Part model, mm, in its own coordinate system. Face numbers are marked on the shaded views. A direction names the side the tool comes from. Round coordinates to 2 decimals unless told otherwise and drop trailing zeros. Use CSV: the item, a comma, the result in double quotes. Start each with the question number.
(1) Drop flat-ended pins along their axis: pin 1 (5 mm diameter, centred on x = 94, z = 2, fed in from +Y); pin 2 (1.5 mm diameter, centred on y = -3, z = 3.5, fed in from +X); pin 3 (1 mm diameter, centred on x = 35, z = 4.5, fed in from -Y). Give the stop position or say it passes through.
(2) Which spindle directions (+Z, -Z, +X, -X, +Y, -Y) get a long thin tool onto all of the face, cutting with end or side? Do the marked faces 1 and 2. Say none if no direction does.
(3) Probe line 1 (X direction, y = -1.75, z = 6.25); line 2 (Y direction, x = 25.5, z = 0.25); line 3 (Y direction, x = 120, z = 0.25). List the from-to ranges inside material, lowest first. Write a range as [from, to].
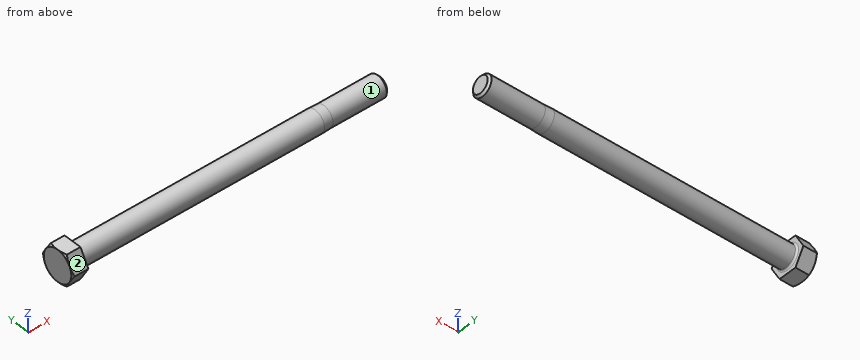
Autodesk Inventor part; units mm, degrees
ref_plane "Work Plane1" through (1.525, 0, 0) normal (0, 0, 1) x (1, 0, 0)
ref_plane "YZ Plane" through (0, 0, 0) normal (1, 0, 0) x (0, 1, 0)
ref_plane "XZ Plane" through (0, 0, 0) normal (0, 1, 0) x (-1, 0, 0)
sketch "Sketch1" plane through (0, 0, 0) normal (0, 0, 1) x (1, 0, 0)
  line L0 (0, 7.1374) -> (0, 4.9276)
  line L1 (114.3, 4.7625) -> (139.7, 4.7625)
  line L2 (139.7, 4.7625) -> (139.7, 0)
  line L3 (139.7, 0) -> (-0.0001, 0)
  line L4 (-27.9401, 0) -> (167.64, 0)
  line L5 (-0.0001, 0) -> (-0.0001, 7.1374)
  line L6 (-0.0001, 7.1374) -> (0, 7.1374)
  line L7 (114.3, 4.7625) -> (110.3312, 4.9276)
  line L8 (110.3312, 4.9276) -> (0, 4.9276)
  line L9 (0, -1.4275) -> (0, 8.5649)
  dimension "d0" = 139.7
  dimension "d1" = 25.4
  dimension "d2" = 9.525
  dimension "d9" = 0.0001
  dimension "d10" = 14.2748
  dimension "d13" = 3.9689
  dimension "d14" = 9.8552
revolve "Body" add sketch "Sketch1" angle 360 about axis through (139.7, 0, 0) along (-1, 0, 0)
sketch "Sketch2" plane through (-0.0001, 0, 0) normal (-1, 0, 0) x (0, 0, 1)
  line L0 (0, 8.2416) -> (7.1374, 4.1208)
  line L1 (7.1374, 4.1208) -> (7.1374, -4.1208)
  line L2 (7.1374, -4.1208) -> (0, -8.2416)
  line L3 (0, -8.2416) -> (-7.1374, -4.1208)
  line L4 (-7.1374, -4.1208) -> (-7.1374, 4.1208)
  line L5 (-7.1374, 4.1208) -> (0, 8.2416)
  point P0 (0, 0)
  point P1 (0, 0)
  dimension "d11" = 14.2748
extrude "Head" add sketch "Sketch2" along normal blind 6.8072
sketch "Sketch4" plane through (0, 0, 0) normal (0, 0, 1) x (1, 0, 0)
  line L0 (-6.8073, 7.1374) -> (-6.8073, 8.2416)
  line L1 (-6.8073, 8.2416) -> (-6.1698, 8.2416)
  line L2 (-6.1698, 8.2416) -> (-6.8073, 7.1374)
  line L3 (-8.1687, 0) -> (1.3613, 0)
  line L4 (-0.0001, 8.2416) -> (-6.8073, 8.2416)
  line L5 (-6.8073, 4.1208) -> (-6.8073, 8.2416)
  dimension "d5" = 30
  dimension "d19" = 14.2748
revolve "Chamfer1" cut sketch "Sketch4" angle 360 about axis through (-10, 0, 0) along (1, 0, 0)
thread "Thread"
chamfer "Chamfer2" distance 0.9739 distance2 0.9447 1 edges at (139.7, -4.7625, 0) measured on face at (139.7, -0.9018, 0.7989)
ref_plane "Work Plane1" through (1.525, 0, 0) normal (0, 0, 1) x (1, 0, 0)
fillet "Fillet2" radius 0.762 1 edges at (0, -4.9276, 0)
equation "\"d0\" = NLG"
equation "\"d1\" = GEL"
equation "\"d2\" = GD"
equation "\"d10\" = SD2"
equation "\"d14\" = BDM"
equation "\"d11\" = SW"
equation "\"d3\" = KOH - SD"
equation "\"d5\" = ANG1"
equation "\"d19\" = SW0"
equation "\"d63\" = R"
equation "\"d15\" = GEL"
equation "\"d6\" = -0.5 * SPD + 0.5 * GD"
equation "\"NLG\" = 139.7"
equation "\"GD\" = NND"
equation "\"BDM\" = 9.8552"
equation "\"KOH\" = 6.8072"
equation "\"GEL\" = 25.4"
equation "\"SW\" = 14.2748"
equation "\"SW0\" = SW"
equation "\"SPD\" = GD1"
equation "\"SD2\" = SW"
equation "\"SD\" = 0"
equation "\"ANG1\" = 30deg"
equation "\"GAL\" = 3.96875"
equation "\"GUL\" = 0.238 * GAL"
equation "\"R\" = 0.762"
equation "\"d62\" = -NLG - SD + GUL"
equation "\"GD1\" = 7.5773"
equation "\"THREADDIA\" = 9.525"
equation "\"TOA\" = 30deg"
equation "\"NND\" = 9.525"
equation "\"E0\" = 1.155 * SW"
properties part number "ANSI/ASME B18.2.1 - 3/8-16 UNC - 5.5" material "Steel, Mild"
Answers:
1,pin 1,"stops at y = 4.93"
1,pin 2,"stops at x = 139.63"
1,pin 3,"stops at y = -2.88"
2,face 1,"+X"
2,face 2,"+Z, +X, -X, -Y"
3,line 1,"x = [-6.81, 0]"
3,line 2,"y = [-4.92, 4.92]"
3,line 3,"y = [-4.76, 4.76]"
